Geometry check sheet. Reference: drawing and pictorial views, mm from the part's lowest x, y, z. A direction names the side the tool comes from. Round coordinates to 2 decimals unless told otherwise and drop trailing zeros. Loops run counter-clockwise (first coordinate to the right, second up) from the corner with the lowest first, then second, coordinate; pieces in that order, holes last. Notation, with made-up numbers: (-3.5, -20.75) - (21.5, -20.75) arc R19 cw to (21.5, 7.25) - close; hole circle Ø1 at (41.5, 31.5). An arc over 180 degrees is marked (long way). Answer as CSV lines item,"result". Start each with the question number.
1) Thickness scan on line 1 along Z through (x, y) = (2, 3); line 2 along Z through (x, y) = (7.5, 12); line 3 along X through (y, z) = (7.25, 19). Record the ranges inside material, lowest first.
2) Cross-section at A-A on y = 3. Record the boundary of the cut face in (x, z).
3) Cross-section at D-D on x = 5.75. Record the boundary of the cut face in (y, z), and give its area (3 significant figures).
4) Access from +Z, -Z, +X, -X, +Y, -Y to the whole of each face (thin tool, end or side, straight path). Record for the marked faces 5, 6 and 7.
5) Cross-section at C-C on z = 32.3. Record the boundary of the cut face in (x, y).
6) Draft check along Y on the marked faces 1, 2, 3 and 4. Enter one of: released by +Y, released by -Y, zero draft, split by the parting line, or undercut.
7) Cross-section at B-B on x = 1. Record the boundary of the cut face in (y, z).
8) Depth check by flat-ended pin: P1, Ø1.5, axis at x = 6.5, y = 9, coming from the -Z side; P2, Ø3, axis at y = 8, z = 7.5, coming from the +X side; P3, Ø8, axis at y = 14, z = 23, coming from the -X side. Enter the tip coordinate at first touch or a pass-through.
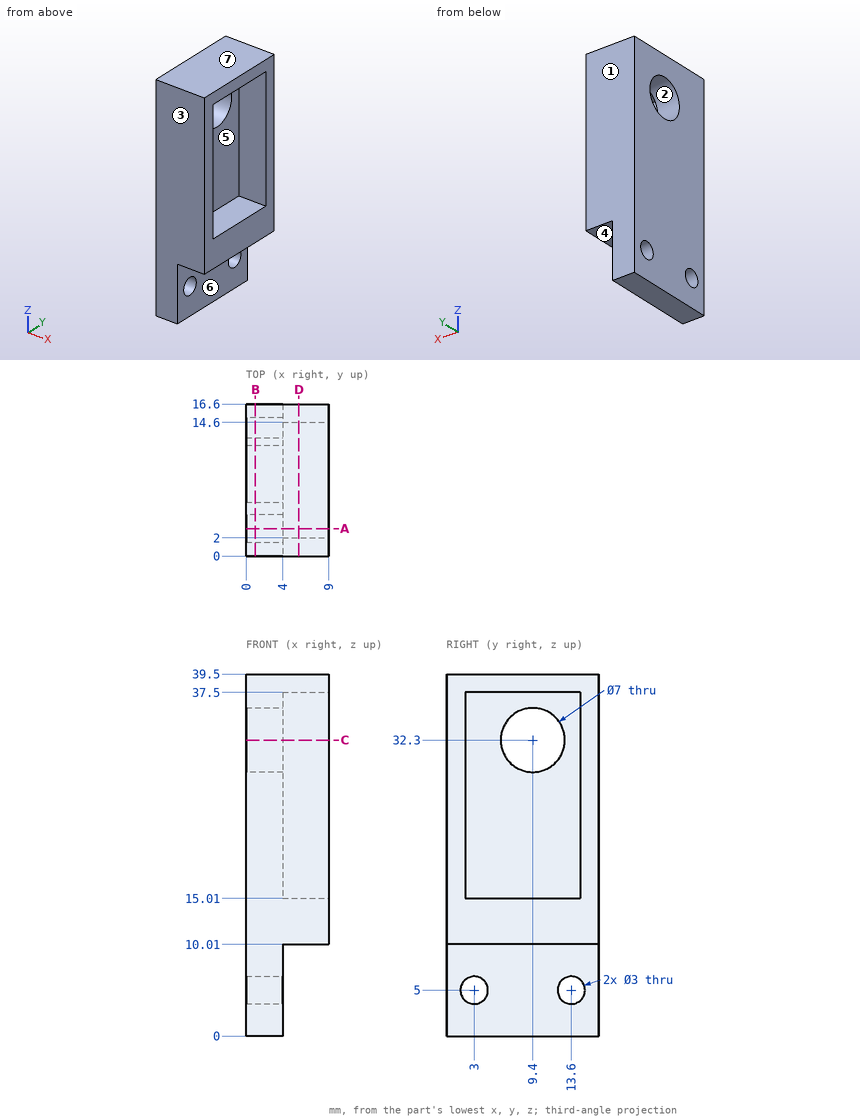
Answer block:
1,line 1,"z = 0 to 3.5, 6.5 to 39.5"
1,line 2,"z = 10.01 to 15.01, 37.5 to 39.5"
1,line 3,"x = 0 to 4"
2,outline,"(0, 0) - (4, 0) - (4, 3.5) - (0, 3.5) - close; (0, 6.5) - (4, 6.5) - (4, 10.01) - (9, 10.01) - (9, 15.01) - (4, 15.01) - (4, 37.5) - (9, 37.5) - (9, 39.5) - (0, 39.5) - close"
3,outline,"(0, 10.01) - (16.6, 10.01) - (16.6, 39.5) - (0, 39.5) - close; hole (2, 15.01) - (14.6, 15.01) - (14.6, 37.5) - (2, 37.5) - close"
3,area,"206 mm^2"
4,face 5,"+X"
4,face 6,"-Z, +X, +Y, -Y"
4,face 7,"+Z, +X, -X, +Y, -Y"
5,outline,"(0, 0) - (9, 0) - (9, 2) - (4, 2) - (4, 5.9) - (0, 5.9) - close; (0, 12.9) - (4, 12.9) - (4, 14.6) - (9, 14.6) - (9, 16.6) - (0, 16.6) - close"
6,face 1,"released by +Y"
6,face 2,"undercut"
6,face 3,"released by -Y"
6,face 4,"zero draft"
7,outline,"(0, 0) - (16.6, 0) - (16.6, 39.5) - (0, 39.5) - close; hole circle Ø3 at (3, 5); hole circle Ø7 at (9.4, 32.3); hole circle Ø3 at (13.6, 5)"
8,P1,"stops at z = 10.01"
8,P2,"stops at x = 4"
8,P3,"stops at x = 0"
